from build123d import *

# Parameters (mm, degrees)
SKETCH_W      = 10
SKETCH_H      = 11.2
SKETCH_W_2    = 15
SKETCH_H_2    = 2
EXTRUDE_DEPTH = 3


with BuildPart() as part:
    # Sketch → Extrude (new body)
    with BuildSketch(Plane.XY):
        with BuildLine():
            Line((40, -6.37), (40, -9.37))
            ThreePointArc((15, -9.37), (27.5, -15.37), (40, -9.37))
            Line((15, -9.37), (15, -6.37))
            Line((15, -6.37), (0, -6.37))
            Line((-3, -6.37), (0, -6.37))
            Line((-3, -0.34), (-3, -6.37))
            Line((-3, -0.34), (0, -0.34))
            Line((0, 14.66), (0, -0.34))
            Line((0, 14.66), (-3, 14.66))
            Line((-3, 14.66), (-3, 20.66))
            Line((-3, 20.66), (0, 20.66))
            Line((0, 20.66), (15, 20.66))
            Line((15, 23.66), (15, 20.66))
            Line((40, 23.66), (15, 23.66))
            Line((40, 20.66), (40, 23.66))
            Line((40, 20.66), (60, 20.66))
            Line((60, 23.66), (60, 20.66))
            Line((85, 23.66), (60, 23.66))
            Line((85, 20.66), (85, 23.66))
            Line((85, 20.66), (100, 20.66))
            Line((100, 20.66), (100, 14.66))
            Line((100, 14.66), (103, 14.66))
            Line((103, 14.66), (103, -0.34))
            Line((103, -0.34), (100, -0.34))
            Line((100, -0.34), (100, -6.37))
            Line((100, -6.37), (85, -6.37))
            Line((85, -6.37), (85, -9.37))
            ThreePointArc((60, -9.37), (72.5, -15.37), (85, -9.37))
            Line((60, -9.37), (60, -6.37))
            Line((60, -6.37), (40, -6.37))
        make_face()
        with Locations((46.64, 7.2)):
            Rectangle(SKETCH_W, SKETCH_H, mode=Mode.SUBTRACT)
        with Locations((62.58, 13.2)):
            Rectangle(SKETCH_W_2, SKETCH_H_2, mode=Mode.SUBTRACT)
    extrude(amount=EXTRUDE_DEPTH)


solid = part.part
Read the model definition and answer for the solid it produces. Units are mm, in the model's axes. A direction names the side the tool comes from. Round coordinates to 2 decimals unless told otherwise and drop trailing zeros. Order: outer loops, then holes, each group sorted by start corner. A loop starts at its lowest first (then second) coordinate and runs counter-clockwise, first axis right, second up.
1) Straight lines are drawn through the part: L1, parallel to X at y = 3, z = 0.25; L2, parallel to Y at x = 1.5, z = 0.25; L3, parallel to X at y = 14.5, z = 2.5. For each, find the intervals that lie inside material, in ascending order.
2) The mould has two halves that part along X. Classify faces 5 (the face through (100, 18, 1)), 6 (the face through (-3, -3, 1)), 7 (the face through (60, -8, 1)), 8 (the face through (93, -6.37, 1)): released by +X, released by -X, zero draft, split by the parting line, or undercut.
3) For faces 1 (the face through (92, 20.66, 1)), 2 (the face through (-1, 14.66, 1)), 3 (the face through (47, 1.6, 1)), 4 (the face through (50, -6.37, 1)), determine the directions among +Z, -Z, +X, -X, +Y, -Y from which every point of the face is accessible in a straight line to the end or side of a thin tool.
4) The part is cut by section B-B on x = 68. Write down the section's boundary in (y, z).
5) The part is cut by section A-A on y = 6. Write down the section's boundary in (x, z).
6) The part is cut by section D-D on z = 1.85. Give the number of separate pieces and of enclosed holes in the cut face, plus the area to 3 significant figures.
7) Flat-ended cylindrical pins translate along their axes: pin 1 (1.5 mm diameter, centred on y = -8, z = 1, fed in from +X); pin 2 (1.6 mm diameter, centred on y = 13, z = 1, fed in from -X); pin 3 (1 mm diameter, centred on x = 48.5, z = 2, fed in from +Y). Find the tip coordinate at first contact, or state that the pin passes through.
8) The part is cut by section C-C on x = 86. Write down the section's boundary in (y, z).
Resolved:
1. L1: x = 0 to 41.64, 51.64 to 103
1. L2: y = -6.37 to 20.66
1. L3: x = 0 to 103
2. face 5: released by +X
2. face 6: released by -X
2. face 7: undercut
2. face 8: zero draft
3. face 1: +Z, -Z, +X, +Y
3. face 2: +Z, -Z, -X
3. face 3: +Z, -Z
3. face 4: +Z, -Z, -Y
4. outline: (-14.73, 0) - (12.2, 0) - (12.2, 3) - (-14.73, 3) - close; (14.2, 0) - (23.66, 0) - (23.66, 3) - (14.2, 3) - close
5. outline: (0, 0) - (41.64, 0) - (41.64, 3) - (0, 3) - close; (51.64, 0) - (103, 0) - (103, 3) - (51.64, 3) - close
6. separate pieces: 1
6. enclosed holes: 2
6. area: 3,150 mm2
7. pin 1: stops at x = 85
7. pin 2: stops at x = 0
7. pin 3: stops at y = 20.66
8. outline: (-6.37, 0) - (20.66, 0) - (20.66, 3) - (-6.37, 3) - close
